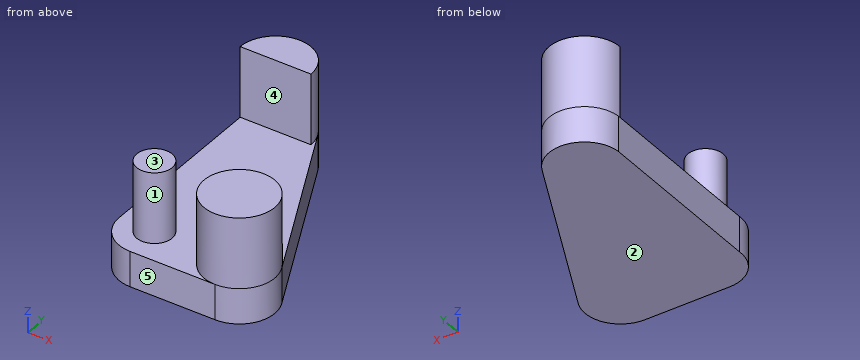
from build123d import *

# Parameters (mm, degrees)
SALIENTE_EXTRUIR1_DEPTH = 5
CROQUIS2_R              = 2.5
CROQUIS2_R_2            = 5
SALIENTE_EXTRUIR2_DEPTH = 10


with BuildPart() as part:
    # Croquis1 → Saliente-Extruir1 (new body)
    with BuildSketch(Plane.XY):
        with BuildLine():
            ThreePointArc((4.507615287, 27.163655338), (-0.972917939, 29.9044297), (-4.992202808, 25.279125636))
            Line((-4.992202808, 25.279125636), (-4.992202808, 24.720874364))
            Line((-4.992202808, 24.720874364), (-4.992202808, 0.279125636))
            ThreePointArc((-4.992202808, 0.279125636), (-3.632879586, -3.435430964), (0, -5))
            Line((0, -5), (12, -5))
            ThreePointArc((12, -5), (16.231918991, -2.662867187), (16.507615287, 2.163655338))
            Line((16.507615287, 2.163655338), (4.507615287, 27.163655338))
        make_face()
    extrude(amount=SALIENTE_EXTRUIR1_DEPTH)

    # Croquis2 → Saliente-Extruir2 (add)
    with BuildSketch(Plane.XY.offset(5)):
        Circle(CROQUIS2_R)
        with Locations(Location((12, 0, 0), (0, 0, 270))):
            Circle(CROQUIS2_R_2)
        with BuildLine():
            Line((-5, 25), (5, 25))
            ThreePointArc((5, 25), (0, 30), (-5, 25))
        make_face()
    extrude(amount=SALIENTE_EXTRUIR2_DEPTH)


solid = part.part
Model file for the job. Use its own axes, mm. Face numbers are marked on the shaded views. A direction names the side the tool comes from. Give positions to 0.01 mm unless a question says otherwise; leave off trailing zeros. Loops run counter-clockwise (first coordinate to the right, second up) from the corner with the lowest first, then second, coordinate; pieces in that order, holes last.
Item 1: Drop flat-ended pins along their axis: P1, Ø1.5, axis at y = 2, z = 9, coming from the -X side; P2, Ø1.5, axis at x = 4, y = 16.5, coming from the +Z side; P3, Ø1.5, axis at y = 9, z = 3.5, coming from the -X side; P4, Ø8, axis at y = 11.5, z = 10.5, coming from the -X side. Give the stop position or say it passes through.
Check values:
P1: stops at x = -2.17
P2: stops at z = 5
P3: stops at x = -4.99
P4: passes through
Item 2: Slice it at D-D (y = 12.5). Write the cut outline in (x, z).
Check values:
outline: (-4.99, 0) - (11.55, 0) - (11.55, 5) - (-4.99, 5) - close
Item 3: Slice it at A-A (x = 14). Write the cut outline in (y, z), plus the area to 3 significant figures.
Check values:
outline: (-4.58, 0) - (7.39, 0) - (7.39, 5) - (4.58, 5) - (4.58, 15) - (-4.58, 15) - close
area: 152 mm2
Item 4: Slice it at C-C (y = -0.5). Write the cut outline in (x, z), plus the area to 3 significant figures.
Check values:
outline: (-4.97, 0) - (16.97, 0) - (16.97, 15) - (7.03, 15) - (7.03, 5) - (2.45, 5) - (2.45, 15) - (-2.45, 15) - (-2.45, 5) - (-4.97, 5) - close
area: 258 mm2
Item 5: Mould opens along Y. For the marked faces 3, 4 and 5 say: +Y half, -Y half, draft (parallel to the pull), parting line (faces both ways), or undercut.
Check values:
face 3: draft
face 4: undercut
face 5: -Y half
Item 6: Which spindle directions (+Z, -Z, +X, -X, +Y, -Y) get a long thin tool onto all of the face, cutting with end or side? Do the marked faces 1 and 2. Say none if no direction does.
Check values:
face 1: +Z
face 2: -Z, +X, -X, +Y, -Y
Item 7: Drill centre lines: line 1 along Z through (x, y) = (2, 23); line 2 along X through (y, z) = (-2, 13); line 3 along Y through (x, z) = (13.5, 10.75). Where is each one in solid material? Low to high.
Check values:
line 1: z = 0 to 5
line 2: x = -1.5 to 1.5, 7.42 to 16.58
line 3: y = -4.77 to 4.77
Item 8: Slice it at B-B (z = 8.75). Write the cut outline in (x, y).
Check values:
outline: (-5, 25) - (5, 25) arc R5 ccw to start; circle Ø5 at (0, 0); circle Ø10 at (12, 0)
